The model under review builds one solid part; all positions refer to its coordinate system, in mm. A direction names the side the tool comes from. Round coordinates to 2 decimals unless told otherwise and drop trailing zeros. Loops run counter-clockwise (first coordinate to the right, second up) from the corner with the lowest first, then second, coordinate; pieces in that order, holes last. Notation, with made-up numbers: M 9.25,-20.5 L 30.25,-20.5 A19 ccw 30.25,3.5 Z; hole C -40,1.5 d5. An arc over 180 degrees is marked long. Return JSON: item names as keys, results as strings. Group by question number.
Q1. Consider section B-B (z = 0). State the section outline as (x, y) points.
Q2. Draft analysis for pull direction Y (two halves, no side actions). For faces 1 (the face through (0, 0, 1)), 2 (the face through (1.299, 11, -2)), 3 (the face through (2.4, 4, -2.2)), state which applies: pulls with the +Y half, pulls with the -Y half, needs draft (parallel to the pull), parting line crosses it, or undercut.
Q3. Consider section C-C (y = 1.5). State the section outline as (x, z) points, and give its area (3 significant figures).
Q4. To check wall thickness, follow line 1 along X through (y, z) = (11, 0); line 2 along X through (y, z) = (0.8, 0); line 3 along Y through (x, z) = (2.5, -0.25). State the ranges of each line that lie inside material, in increasing order.
Q5. Consider section A-A (y = 7). State the section outline as (x, z) points, and give its area (3 significant figures).
Q6. Consider section D-D (x = 4). State the section outline as (y, z) points.
Q7. Clearance check with flat-ended pins moving along their axes: pin 1 Ø2.5 at (x, z) = (-3, -1.5) entering from +Y; pin 2 Ø5 at (x, y) = (4, 9) entering from -Z; pin 3 Ø2 at (y, z) = (13, -2) entering from -X. State where each tip first meets the part, or that it passes through.
Q8. For faces 4 (the face through (0, 19, 3)), 5 (the face through (-0.098, 2.986, 1.756)), 6 (the face through (5, 22, -2)), list the 3-axis set-ups (+Z, -Z, +X, -X, +Y, -Y) from which the entire face can be reached by the end or side of a thin tool; tool diameter is ignored.
from build123d import *

# Parameters (mm, degrees)
SKETCH1_R           = 7
BOSS_EXTRUDE1_DEPTH = 22
CAVITY1_START       = 2
CAVITY1_OUTLINE_R   = 5
CAVITY1_DEPTH       = 20
CAVITY1_START_2     = 19
CAVITY1_2_DEPTH     = 3
CAVITY1_3_OUTLINE_R = 0.75
CAVITY1_3_DEPTH     = 2
SKETCH2_R           = 0.5
CUT_EXTRUDE1_DEPTH  = 23.315913604


# Read off the part's stored shape, not the designer's step: Cavity1
with BuildPart() as part:
    # Sketch1 → Boss-Extrude1 (new body)
    with BuildSketch(Plane(origin=(0, 0, 0), x_dir=(1, 0, 0), z_dir=(0, 1, 0))):
        with Locations(Location((0, 0, 0), (0, 0, 270))):
            Circle(SKETCH1_R)
    extrude(amount=BOSS_EXTRUDE1_DEPTH)

    # Cavity1 outline → Cavity1 (cut)
    with BuildSketch(Plane(origin=(0, 0, 0), x_dir=(1, 0, 0), z_dir=(0, 1, 0)).offset(CAVITY1_START)):
        Circle(CAVITY1_OUTLINE_R)
        with BuildLine():
            Line((0, -1.5), (2.165063509, -2.75))
            ThreePointArc((2.165063509, -2.75), (0, -3.5), (-2.165063509, -2.75))
            Line((-2.165063509, -2.75), (0, -1.5))
        make_face(mode=Mode.SUBTRACT)
        with BuildLine():
            Line((-1.299038106, 0.75), (-3.464101615, -0.5))
            ThreePointArc((-3.464101615, -0.5), (-3.031088913, 1.75), (-1.299038106, 3.25))
            Line((-1.299038106, 3.25), (-1.299038106, 0.75))
        make_face(mode=Mode.SUBTRACT)
        with BuildLine():
            Line((3.464101615, -0.5), (1.299038106, 0.75))
            Line((1.299038106, 0.75), (1.299038106, 3.25))
            ThreePointArc((1.299038106, 3.25), (3.031088913, 1.75), (3.464101615, -0.5))
        make_face(mode=Mode.SUBTRACT)
    extrude(amount=CAVITY1_DEPTH, mode=Mode.SUBTRACT)

    # Cavity1 2 outline → Cavity1 2 (cut)
    with BuildSketch(Plane(origin=(0, 0, 0), x_dir=(1, 0, 0), z_dir=(0, 1, 0)).offset(CAVITY1_START_2)):
        with BuildLine():
            Line((1.299038106, 3.25), (1.299038106, 0.75))
            Line((1.299038106, 0.75), (3.464101615, -0.5))
            ThreePointArc((3.464101615, -0.5), (3.031088913, 1.75), (1.299038106, 3.25))
        make_face()
        with BuildLine():
            ThreePointArc((-1.299038106, 3.25), (-3.031088913, 1.75), (-3.464101615, -0.5))
            Line((-3.464101615, -0.5), (-1.299038106, 0.75))
            Line((-1.299038106, 0.75), (-1.299038106, 3.25))
        make_face()
        with BuildLine():
            ThreePointArc((-2.165063509, -2.75), (0, -3.5), (2.165063509, -2.75))
            Line((2.165063509, -2.75), (0, -1.5))
            Line((0, -1.5), (-2.165063509, -2.75))
        make_face()
    extrude(amount=CAVITY1_2_DEPTH, mode=Mode.SUBTRACT)

    # Cavity1 3 outline → Cavity1 3 (cut)
    # profile 1 of 3: a face of its own
    with BuildSketch(Plane(origin=(0, 0, 0), x_dir=(1, 0, 0), z_dir=(0, 1, 0)).offset(CAVITY1_START)):
        with BuildLine():
            Line((1.299038106, 3.25), (1.299038106, 0.75))
            Line((1.299038106, 0.75), (3.464101615, -0.5))
            ThreePointArc((3.464101615, -0.5), (3.031088913, 1.75), (1.299038106, 3.25))
        make_face()
        with Locations((2.165063509, 1.25)):
            Circle(CAVITY1_3_OUTLINE_R, mode=Mode.SUBTRACT)
    # profile 2 of 3: a face of its own
    with BuildSketch(Plane(origin=(0, 0, 0), x_dir=(1, 0, 0), z_dir=(0, 1, 0)).offset(CAVITY1_START)):
        with BuildLine():
            ThreePointArc((-1.299038106, 3.25), (-3.031088913, 1.75), (-3.464101615, -0.5))
            Line((-3.464101615, -0.5), (-1.299038106, 0.75))
            Line((-1.299038106, 0.75), (-1.299038106, 3.25))
        make_face()
        with Locations((-2.165063509, 1.25)):
            Circle(CAVITY1_3_OUTLINE_R, mode=Mode.SUBTRACT)
    # profile 3 of 3: a face of its own
    with BuildSketch(Plane(origin=(0, 0, 0), x_dir=(1, 0, 0), z_dir=(0, 1, 0)).offset(CAVITY1_START)):
        with BuildLine():
            ThreePointArc((-2.165063509, -2.75), (0, -3.5), (2.165063509, -2.75))
            Line((2.165063509, -2.75), (0, -1.5))
            Line((0, -1.5), (-2.165063509, -2.75))
        make_face()
        with Locations((0, -2.5)):
            Circle(CAVITY1_3_OUTLINE_R, mode=Mode.SUBTRACT)
    extrude(amount=CAVITY1_3_DEPTH, mode=Mode.SUBTRACT)

    # Sketch2 → Cut-Extrude1 (cut, through all)
    with BuildSketch(Plane(origin=(0, 2, 0), x_dir=(1, 0, 0), z_dir=(0, 1, 0))):
        with Locations(Location((0, 0, 0), (0, 0, 270))):
            Circle(SKETCH2_R)
    extrude(amount=-CUT_EXTRUDE1_DEPTH, mode=Mode.SUBTRACT)


solid = part.part
Values:
{
 "1": {"outline": "M -7,0 L -0.5,0 L -0.5,2 L -5,2 L -5,22 L -7,22 Z; M -3.5,4 L -2.6,4 L -2.6,19 L -3.5,19 Z; M 0.5,0 L 7,0 L 7,22 L 5,22 L 5,2 L 0.5,2 Z; M 2.6,4 L 3.5,4 L 3.5,19 L 2.6,19 Z"},
 "2": {"face 1": "pulls with the -Y half", "face 2": "needs draft", "face 3": "undercut"},
 "3": {"outline": "C 0,0 d14; hole C 0,0 d1", "area": "153 mm2"},
 "4": {"line 1": "x = -7 to -5, -3.5 to -2.6, 2.6 to 3.5, 5 to 7", "line 2": "x = -7 to -0.5, 0.5 to 7", "line 3": "y = 0 to 2, 4 to 19"},
 "5": {"outline": "C 0,0 d14; M -3.46,0.5 A3.5 ccw -1.3,-3.25 L -1.3,-0.75 Z; M -2.17,2.75 L 0,1.5 L 2.17,2.75 A3.5 ccw Z; M 1.3,-3.25 A3.5 ccw 3.46,0.5 L 1.3,-0.75 Z; hole C 0,0 d10", "area": "90.2 mm2"},
 "6": {"outline": "M 0,-5.74 L 22,-5.74 L 22,-3 L 2,-3 L 2,3 L 22,3 L 22,5.74 L 0,5.74 Z"},
 "7": {"pin 1": "stops at y = 19", "pin 2": "stops at z = -6.84", "pin 3": "stops at x = -6.93"},
 "8": {"face 4": "+Y", "face 5": "none", "face 6": "+Z, -Z, +X, -X, +Y"}
}
